from build123d import *

# Parameters (mm, degrees)
F2_R     = 6.5
F2_R_2   = 5.75
F3_DEPTH = 1
F4_W     = 6
F4_H     = 2
F5_DEPTH = 3
F5_TAPER = 10


with BuildPart() as f1:
    # F0 (on Right) → F1 (revolve)
    with BuildSketch(Plane.YZ):
        Polygon((0, 8), (0, 0), (3.5, 0), (3.85, 2), (3.85, 7), (6.5, 7), (6.5, 8), align=None)
    revolve(axis=Axis((0, 0, 6.5057562609), (0, 0, 1)))

    # F2 (on face) → F3 (join)
    with BuildSketch(Plane(origin=(0, 0, 7), x_dir=(1, 0, 0), z_dir=(0, 0, -1))):
        Circle(F2_R)
        Circle(F2_R_2, mode=Mode.SUBTRACT)
    extrude(amount=F3_DEPTH)

    # F4 (on face) → F5 (cut)
    with BuildSketch(Plane.XY.offset(8)):
        Rectangle(F4_W, F4_H)
    extrude(amount=-F5_DEPTH, taper=F5_TAPER, mode=Mode.SUBTRACT)


solid = f1.part
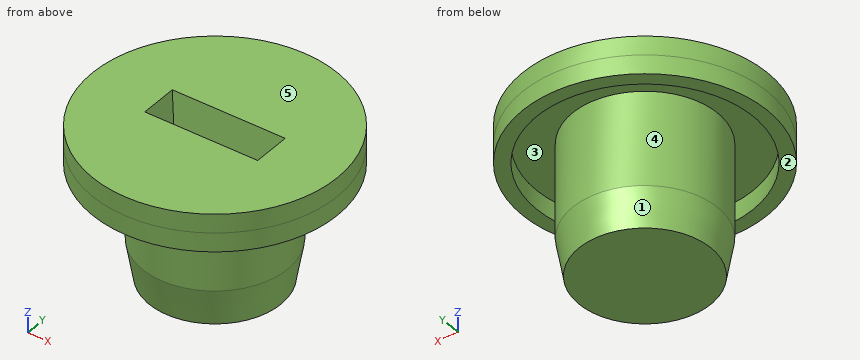
Read the model definition and answer for the solid it produces. Units are mm, in the model's axes. Face numbers are marked on the shaded views. A direction names the side the tool comes from. Round coordinates to 2 decimals unless told otherwise and drop trailing zeros. Write each loop counter-clockwise with the first axis right and the second up, starting at its lowest first coordinate (ties: lowest second). Pieces come first, ordered by that corner, then holes.
1. Straight lines are drawn through the part: L1, parallel to X at y = 0, z = 6.4; L2, parallel to Y at x = 0, z = 6.65; L3, parallel to Y at x = 0, z = 6.2. For each, find the intervals that lie inside material, in ascending order.
2. The part is cut by section D-D, the plane z = 0.5. Determine the outline of the cut face in (x, y) (1 decimal), then the cut area to 3 significant figures.
3. Determine the mould class of the marked faces 1, 2 and 3 for opening direction X: pulls with the +X half, pulls with the -X half, needs draft (parallel to the pull), parting line crosses it, or undercut.
4. Which of the six approach directions +Z, -Z, +X, -X, +Y, -Y give full straight-line access (tool end or side, diameter ignored) to the marked faces 4 and 5?
5. The part is cut by section B-B, the plane y = -5.5. Determine the outline of the cut face in (x, z), then the cut area to 3 significant figures.
6. The part is cut by section A-A, the plane x = -5.25. Determine the outline of the cut face in (y, z).
7. The part is cut by section C-C, the plane z = 4.5. Determine the outline of the cut face in (x, y).
8. Given pin 1 Ø1 at (x, z) = (-0.5, 2) entering from +Y; pin 2 Ø0.5 at (x, y) = (-1, 0) entering from +Z; pin 3 Ø1 at (y, z) = (-4, 6.5) entering from -X, each flat-ended and moving along its own axis, determine where each tip first touches the part or whether it passes through.
Values:
1. L1: x = -6.5 to -5.75, -3.85 to -2.72, 2.72 to 3.85, 5.75 to 6.5
1. L2: y = -6.5 to -5.75, -3.85 to -0.76, 0.76 to 3.85, 5.75 to 6.5
1. L3: y = -6.5 to -5.75, -3.85 to -0.68, 0.68 to 3.85, 5.75 to 6.5
2. outline: circle Ø7.2 at (0, 0)
2. area: 40.4 mm2
3. face 1: parting line crosses it
3. face 2: needs draft
3. face 3: undercut
4. face 4: -Z
4. face 5: +Z, +X, -X, +Y, -Y
5. outline: (-3.46, 6) - (-1.68, 6) - (-1.68, 7) - (1.68, 7) - (1.68, 6) - (3.46, 6) - (3.46, 8) - (-3.46, 8) - close
5. area: 10.5 mm2
6. outline: (-3.83, 6) - (-2.35, 6) - (-2.35, 7) - (2.35, 7) - (2.35, 6) - (3.83, 6) - (3.83, 8) - (-3.83, 8) - close
7. outline: circle Ø7.7 at (0, 0)
8. pin 1: stops at y = 3.85
8. pin 2: stops at z = 5
8. pin 3: stops at x = -5.48
